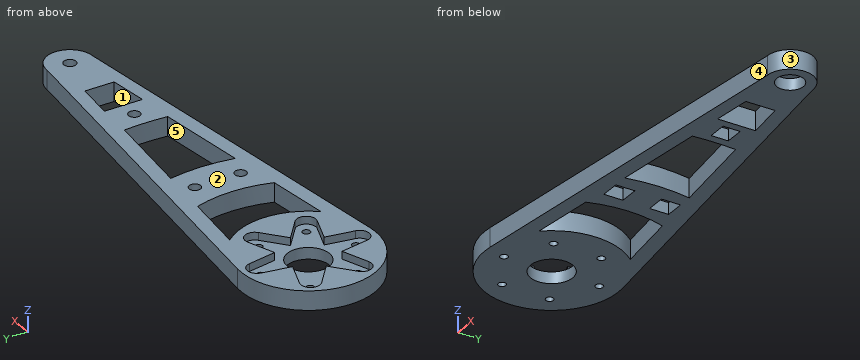
```python
from build123d import *

# Parameters (mm, degrees)
F0_R     = 1.6
F0_R_2   = 5.5
F1_DEPTH = 3
F2_DEPTH = 5
F3_R     = 1
F3_W     = 5
F3_H     = 5
F3_H_2   = 4.5
F3_R_2   = 3.5
F4_DEPTH = 3
F5_R     = 1.5
F6_DEPTH = 25
F7_DEPTH = 25


# Not quite as in the source:
# - a feature names something its author has since deleted; it is built from what else it names


with BuildPart() as f1:
    # F0 (on Top) → F1 (new body)
    with BuildSketch(Plane.XY):
        with BuildLine():
            Line((100.0328712093, 5.9999099563), (2.0188625271, 17.3831583464))
            ThreePointArc((2.0188625271, 17.3831583464), (-17.5, 0), (2.0188625271, -17.3831583464))
            Line((2.0188625271, -17.3831583464), (100.0328712093, -5.9999099563))
            ThreePointArc((100.0328712093, -5.9999099563), (106, 0), (100.0328712093, 5.9999099563))
        make_face()
        with BuildLine():
            ThreePointArc((-2.4633505863, 13.9265019214), (0, 16), (2.4633505863, 13.9265019214))
            Line((2.4633505863, 13.9265019214), (3.75, 6.4951905284))
            Line((3.75, 6.4951905284), (10.8290291566, 9.0965751469))
            ThreePointArc((10.8290291566, 9.0965751469), (13.8564064606, 8), (13.2923797429, 4.8299267745))
            Line((13.2923797429, 4.8299267745), (7.5, 0))
            Line((7.5, 0), (13.2923797429, -4.8299267745))
            ThreePointArc((13.2923797429, -4.8299267745), (13.8564064606, -8), (10.8290291566, -9.0965751469))
            Line((10.8290291566, -9.0965751469), (3.75, -6.4951905284))
            Line((3.75, -6.4951905284), (2.4633505863, -13.9265019214))
            ThreePointArc((2.4633505863, -13.9265019214), (0, -16), (-2.4633505863, -13.9265019214))
            Line((-2.4633505863, -13.9265019214), (-3.75, -6.4951905284))
            Line((-3.75, -6.4951905284), (-10.8290291566, -9.0965751469))
            ThreePointArc((-10.8290291566, -9.0965751469), (-13.8564064606, -8), (-13.2923797429, -4.8299267745))
            Line((-13.2923797429, -4.8299267745), (-7.5, 0))
            Line((-7.5, 0), (-13.2923797429, 4.8299267745))
            ThreePointArc((-13.2923797429, 4.8299267745), (-13.8564064606, 8), (-10.8290291566, 9.0965751469))
            Line((-10.8290291566, 9.0965751469), (-3.75, 6.4951905284))
            Line((-3.75, 6.4951905284), (-2.4633505863, 13.9265019214))
        make_face(mode=Mode.SUBTRACT)
        with BuildLine():
            Line((30.3766267594, -10.0628299558), (13.8329335508, -11.9841978461))
            ThreePointArc((13.8329335508, -11.9841978461), (18.3022143096, 0), (13.8329335508, 11.9841978461))
            Line((13.8329335508, 11.9841978461), (30.3766267594, 10.0628299558))
            ThreePointArc((30.3766267594, 10.0628299558), (32, 0), (30.3766267594, -10.0628299558))
        make_face(mode=Mode.SUBTRACT)
        with BuildLine():
            Line((68.0861847768, -5.6832798143), (44.198061298, -8.4576224495))
            ThreePointArc((44.198061298, -8.4576224495), (45, 0), (44.198061298, 8.4576224495))
            Line((44.198061298, 8.4576224495), (68.0861847768, 5.6832798143))
            ThreePointArc((68.0861847768, 5.6832798143), (68.3229699802, 0), (68.0861847768, -5.6832798143))
        make_face(mode=Mode.SUBTRACT)
        Polygon((77.5869291791, -5), (77.5869291791, 5), (87.5869291791, 3.8386100576), (87.5869291791, -3.8386100576), align=None, mode=Mode.SUBTRACT)
        with Locations((100, 0)):
            Circle(F0_R, mode=Mode.SUBTRACT)
        with BuildLine():
            Line((3.75, 6.4951905284), (2.4633505863, 13.9265019214))
            ThreePointArc((2.4633505863, 13.9265019214), (0, 16), (-2.4633505863, 13.9265019214))
            Line((-2.4633505863, 13.9265019214), (-3.75, 6.4951905284))
            Line((-3.75, 6.4951905284), (-10.8290291566, 9.0965751469))
            ThreePointArc((-10.8290291566, 9.0965751469), (-13.8564064606, 8), (-13.2923797429, 4.8299267745))
            Line((-13.2923797429, 4.8299267745), (-7.5, 0))
            Line((-7.5, 0), (-13.2923797429, -4.8299267745))
            ThreePointArc((-13.2923797429, -4.8299267745), (-13.8564064606, -8), (-10.8290291566, -9.0965751469))
            Line((-10.8290291566, -9.0965751469), (-3.75, -6.4951905284))
            Line((-3.75, -6.4951905284), (-2.4633505863, -13.9265019214))
            ThreePointArc((-2.4633505863, -13.9265019214), (0, -16), (2.4633505863, -13.9265019214))
            Line((2.4633505863, -13.9265019214), (3.75, -6.4951905284))
            Line((3.75, -6.4951905284), (10.8290291566, -9.0965751469))
            ThreePointArc((10.8290291566, -9.0965751469), (13.8564064606, -8), (13.2923797429, -4.8299267745))
            Line((13.2923797429, -4.8299267745), (7.5, 0))
            Line((7.5, 0), (13.2923797429, 4.8299267745))
            ThreePointArc((13.2923797429, 4.8299267745), (13.8564064606, 8), (10.8290291566, 9.0965751469))
            Line((10.8290291566, 9.0965751469), (3.75, 6.4951905284))
        make_face()
        Circle(F0_R_2, mode=Mode.SUBTRACT)
    extrude(amount=F1_DEPTH)

    # F0 (on Top) → F2 (join)
    with BuildSketch(Plane.XY):
        with BuildLine():
            Line((100.0328712093, 5.9999099563), (2.0188625271, 17.3831583464))
            ThreePointArc((2.0188625271, 17.3831583464), (-17.5, 0), (2.0188625271, -17.3831583464))
            Line((2.0188625271, -17.3831583464), (100.0328712093, -5.9999099563))
            ThreePointArc((100.0328712093, -5.9999099563), (106, 0), (100.0328712093, 5.9999099563))
        make_face()
        with BuildLine():
            ThreePointArc((-2.4633505863, 13.9265019214), (0, 16), (2.4633505863, 13.9265019214))
            Line((2.4633505863, 13.9265019214), (3.75, 6.4951905284))
            Line((3.75, 6.4951905284), (10.8290291566, 9.0965751469))
            ThreePointArc((10.8290291566, 9.0965751469), (13.8564064606, 8), (13.2923797429, 4.8299267745))
            Line((13.2923797429, 4.8299267745), (7.5, 0))
            Line((7.5, 0), (13.2923797429, -4.8299267745))
            ThreePointArc((13.2923797429, -4.8299267745), (13.8564064606, -8), (10.8290291566, -9.0965751469))
            Line((10.8290291566, -9.0965751469), (3.75, -6.4951905284))
            Line((3.75, -6.4951905284), (2.4633505863, -13.9265019214))
            ThreePointArc((2.4633505863, -13.9265019214), (0, -16), (-2.4633505863, -13.9265019214))
            Line((-2.4633505863, -13.9265019214), (-3.75, -6.4951905284))
            Line((-3.75, -6.4951905284), (-10.8290291566, -9.0965751469))
            ThreePointArc((-10.8290291566, -9.0965751469), (-13.8564064606, -8), (-13.2923797429, -4.8299267745))
            Line((-13.2923797429, -4.8299267745), (-7.5, 0))
            Line((-7.5, 0), (-13.2923797429, 4.8299267745))
            ThreePointArc((-13.2923797429, 4.8299267745), (-13.8564064606, 8), (-10.8290291566, 9.0965751469))
            Line((-10.8290291566, 9.0965751469), (-3.75, 6.4951905284))
            Line((-3.75, 6.4951905284), (-2.4633505863, 13.9265019214))
        make_face(mode=Mode.SUBTRACT)
        with BuildLine():
            Line((30.3766267594, -10.0628299558), (13.8329335508, -11.9841978461))
            ThreePointArc((13.8329335508, -11.9841978461), (18.3022143096, 0), (13.8329335508, 11.9841978461))
            Line((13.8329335508, 11.9841978461), (30.3766267594, 10.0628299558))
            ThreePointArc((30.3766267594, 10.0628299558), (32, 0), (30.3766267594, -10.0628299558))
        make_face(mode=Mode.SUBTRACT)
        with BuildLine():
            Line((68.0861847768, -5.6832798143), (44.198061298, -8.4576224495))
            ThreePointArc((44.198061298, -8.4576224495), (45, 0), (44.198061298, 8.4576224495))
            Line((44.198061298, 8.4576224495), (68.0861847768, 5.6832798143))
            ThreePointArc((68.0861847768, 5.6832798143), (68.3229699802, 0), (68.0861847768, -5.6832798143))
        make_face(mode=Mode.SUBTRACT)
        Polygon((77.5869291791, -5), (77.5869291791, 5), (87.5869291791, 3.8386100576), (87.5869291791, -3.8386100576), align=None, mode=Mode.SUBTRACT)
        with Locations((100, 0)):
            Circle(F0_R, mode=Mode.SUBTRACT)
    extrude(amount=F2_DEPTH)

    # F3 (on face) → F4 (cut)
    with BuildSketch(Plane.XY):
        with Locations((0, -12.5)):
            Circle(F3_R)
        with Locations((10.8253175473, -6.25)):
            Circle(F3_R)
        with Locations((10.8253175473, 6.25)):
            Circle(F3_R)
        with Locations((0, 12.5)):
            Circle(F3_R)
        with Locations((-10.8253175473, 6.25)):
            Circle(F3_R)
        with Locations((-10.8253175473, -6.25)):
            Circle(F3_R)
        with Locations((38, 6)):
            Rectangle(F3_W, F3_H)
        with Locations((73, 0)):
            Rectangle(F3_W, F3_H_2)
        with Locations((38, -6)):
            Rectangle(F3_W, F3_H)
        with Locations((100.0133901834, 0)):
            Circle(F3_R_2)
    extrude(amount=F4_DEPTH, mode=Mode.SUBTRACT)

    # F5 (on face) → F6 (cut)
    with BuildSketch(Plane.XY):
        with Locations((38, -6)):
            Circle(F5_R)
        with Locations((73, 0)):
            Circle(F5_R)
        with Locations((38, 6)):
            Circle(F5_R)
    extrude(amount=F6_DEPTH, mode=Mode.SUBTRACT)

    # F3 (on face) → F7 (cut)
    with BuildSketch(Plane.XY):
        with Locations((0, -12.5)):
            Circle(F3_R)
        with Locations((10.8253175473, -6.25)):
            Circle(F3_R)
        with Locations((10.8253175473, 6.25)):
            Circle(F3_R)
        with Locations((0, 12.5)):
            Circle(F3_R)
        with Locations((-10.8253175473, 6.25)):
            Circle(F3_R)
        with Locations((-10.8253175473, -6.25)):
            Circle(F3_R)
        with Locations((73, 0)):
            Rectangle(F3_W, F3_H_2)
    extrude(amount=-F7_DEPTH, mode=Mode.SUBTRACT)


solid = f1.part
```
Input: part model. Units: mm. Frame: model coordinates. Face numbers are marked on the shaded views. A direction names the side the tool comes from. Round coordinates to 2 decimals unless told otherwise and drop trailing zeros. Loops run counter-clockwise (first coordinate to the right, second up) from the corner with the lowest first, then second, coordinate; pieces in that order, holes last. Notation, with made-up numbers: (1, 26) - (39, 26) arc R28 cw to (39, 45) - close; hole circle Ø4 at (-34.75, 51.25). An arc over 180 degrees is marked (long way). One line per item, written item: value. Start each with the question number.
(1) Section A-A, the plane x = 83. Return loops of the section in (y, z), plus the area to 3 significant figures.
(2) Access query for the marked faces 4 and 5. Directions: +Z, -Z, +X, -X, +Y, -Y. A direction counts if a zero-diameter tool reaches every point of the face in a straight line with its end or side. Return the directions, or none.
(3) Section C-C, the plane z = 2.2. Count the separate pieces of the cut face and the enclosed holes in it, plus the area to 3 significant figures.
(4) Ray query, line 1 (Y direction, x = 0, z = 0.85); line 2 (Y direction, x = 100, z = 3.5); line 3 (X direction, y = 2.5, z = 4.25). Return the intervals inside material, ascending. Write a range as [from, to].
(5) Draft query along Y for the marked faces 1, 2 and 3. Return one class per face: +Y half, -Y half, draft (parallel to the pull), parting line (faces both ways), or undercut.
(6) Contact query for flat-ended pins moving along their axis: P1, Ø3.5, axis at x = 73, y = 0, coming from the -Z side; P2, Ø0.9, axis at y = 1, z = 2, coming from the +X side; P3, Ø1.5, axis at x = -2.5, z = 1, coming from the +Y side. Output: stop coordinate, or through.
(7) Section B-B, the plane x = 38. Return loops of the section in (y, z).
Results below:
1. outline: (-7.98, 0) - (-4.37, 0) - (-4.37, 5) - (-7.98, 5) - close; (4.37, 0) - (7.98, 0) - (7.98, 5) - (4.37, 5) - close
1. area: 36.1 mm^2
2. face 4: +Z, -Z, +X, -Y
2. face 5: +Z, -Z
3. separate pieces: 1
3. enclosed holes: 14
3. area: 1,940 mm^2
4. line 1: [-17.5, -13.5], [-11.5, -5.5], [5.5, 11.5], [13.5, 17.5]
4. line 2: [-6, -1.6], [1.6, 6]
4. line 3: [-17.32, -10.5], [10.5, 18.13], [31.9, 44.93], [68.28, 77.59], [87.59, 105.45]
5. face 1: undercut
5. face 2: draft
5. face 3: parting line
6. P1: z = 3
6. P2: x = 105.97
6. P3: y = 17.41
7. outline: (-13.2, 0) - (-8.5, 0) - (-8.5, 3) - (-7.5, 3) - (-7.5, 5) - (-13.2, 5) - close; (-4.5, 3) - (-3.5, 3) - (-3.5, 0) - (3.5, 0) - (3.5, 3) - (4.5, 3) - (4.5, 5) - (-4.5, 5) - close; (7.5, 3) - (8.5, 3) - (8.5, 0) - (13.2, 0) - (13.2, 5) - (7.5, 5) - close
